Geometry check sheet. Reference: the model listing, model coordinates, mm. Face numbers are marked on the shaded views. A direction names the side the tool comes from. Round coordinates to 2 decimals unless told otherwise and drop trailing zeros. Write each loop counter-clockwise with the first axis right and the second up, starting at its lowest first coordinate (ties: lowest second). Pieces come first, ordered by that corner, then holes. Notation, with made-up numbers: (14, 62) -> (19, 62) arc R25 cw to (19, 88) -> close; hole circle Ø4 at (-11, 49.5). An arc over 180 degrees is marked (long way). Use a Markdown table: item, result.
```python
from build123d import *

# Parameters (mm, degrees)
F0_R          = 14
F1_DEPTH      = 10
F1_DEPTH_BACK = 10
F2_R          = 5
F3_R          = 5
F4_R          = 1
F5_DEPTH      = 25
F6_R          = 5


with BuildPart() as f1:
    # F0 (on Top) → F1 (new body, two sides)
    with BuildSketch(Plane.XY) as f1_sk:
        with BuildLine():
            ThreePointArc((-14.1332940251, -7.5), (3.86440782, -15.5263116097), (16, 0))
            ThreePointArc((16, 0), (3.86440782, 15.5263116097), (-14.1332940251, 7.5))
            ThreePointArc((-14.1332940251, 7.5), (-14.6133919535, 6.5152724896), (-15.0249792013, 5.5))
            ThreePointArc((-15.0249792013, 5.5), (-16, 0), (-15.0249792013, -5.5))
            ThreePointArc((-15.0249792013, -5.5), (-14.6133919535, -6.5152724896), (-14.1332940251, -7.5))
        make_face()
        Circle(F0_R, mode=Mode.SUBTRACT)
        with BuildLine():
            ThreePointArc((-15.0249792013, 5.5), (-14.6133919535, 6.5152724896), (-14.1332940251, 7.5))
            Line((-14.1332940251, 7.5), (-58.6950893998, 7.5))
            Line((-58.6950893998, 7.5), (-58.6950893998, 40))
            Line((-58.6950893998, 40), (-60.6950893998, 40))
            Line((-60.6950893998, 40), (-60.6950893998, -40))
            Line((-60.6950893998, -40), (-58.6950893998, -40))
            Line((-58.6950893998, -40), (-58.6950893998, -7.5))
            Line((-58.6950893998, -7.5), (-14.1332940251, -7.5))
            ThreePointArc((-14.1332940251, -7.5), (-14.6133919535, -6.5152724896), (-15.0249792013, -5.5))
            Line((-15.0249792013, -5.5), (-58.6950893998, -5.5))
            Line((-58.6950893998, -5.5), (-58.6950893998, 5.5))
            Line((-58.6950893998, 5.5), (-15.0249792013, 5.5))
        make_face()
    extrude(amount=F1_DEPTH)
    extrude(f1_sk.sketch, amount=-F1_DEPTH_BACK)

    # F2
    f2_edges = [f1.edges().sort_by_distance(p)[0] for p in [
        (-14.133294, -7.5, 0),
        (-15.024979, -5.5, 0),
        (-15.024979, 5.5, 0),
        (-14.133294, 7.5, 0),
    ]]
    fillet(f2_edges, radius=F2_R)

    # F3
    f3_edges = [f1.edges().sort_by_distance(p)[0] for p in [
        (-58.695089, -5.5, 0),
        (-58.695089, 5.5, 0),
    ]]
    fillet(f3_edges, radius=F3_R)

    # F4 (on face) → F5 (cut)
    with BuildSketch(Plane.XY.offset(10)):
        with Locations((-15.1501176879, -5.7808761485)):
            Circle(F4_R)
        with Locations((-15.2443397102, 5.5276307583)):
            Circle(F4_R)
    extrude(amount=-F5_DEPTH, mode=Mode.SUBTRACT)

    # F6
    f6_edges = [f1.edges().sort_by_distance(p)[0] for p in [
        (-58.695089, 7.5, 0),
    ]]
    fillet(f6_edges, radius=F6_R)


solid = f1.part
```
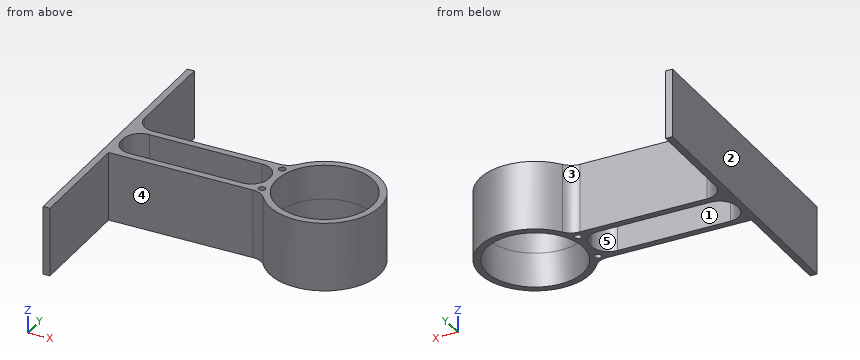
(1) Section check A-A on x = -43. Record the cut outline in (y, z).
A:
| item | result |
|---|---|
| outline | (-7.5, -10) -> (-5.5, -10) -> (-5.5, 10) -> (-7.5, 10) -> close; (5.5, -10) -> (7.5, -10) -> (7.5, 10) -> (5.5, 10) -> close |
(2) Section check C-C on x = -10.5. Record the cut outline in (y, z).
A:
| item | result |
|---|---|
| outline | (-12.07, -10) -> (-9.26, -10) -> (-9.26, 10) -> (-12.07, 10) -> close; (9.26, -10) -> (12.07, -10) -> (12.07, 10) -> (9.26, 10) -> close |
(3) Release check for a two-part mould opening along X. For the marked faces 1 and 2 record: +X half, -X half, draft (parallel to the pull), parting line (faces both ways), or undercut.
A:
| item | result |
|---|---|
| face 1 | undercut |
| face 2 | -X half |
(4) Section check B-B on z = -4. Record the cut outline in (x, y), plus the area to 3 significant figures.
A:
| item | result |
|---|---|
| outline | (-60.7, -40) -> (-58.7, -40) -> (-58.7, -7.5) -> (-16.87, -7.5) arc R5 cw to (-12.86, -9.52) arc R16 ccw (long way) to (-12.86, 9.52) arc R5 cw to (-16.87, 7.5) -> (-53.7, 7.5) arc R5 cw to (-58.7, 12.5) -> (-58.7, 40) -> (-60.7, 40) -> close; hole (-58.7, -0.5) arc R5 ccw to (-53.7, -5.5) -> (-20.99, -5.5) arc R5 ccw to (-16, -0.38) arc R16 cw to (-16, 0.38) arc R5 ccw to (-20.99, 5.5) -> (-53.7, 5.5) arc R5 ccw to (-58.7, 0.5) -> close; hole circle Ø2 at (-15.24, 5.53); hole circle Ø2 at (-15.15, -5.78); hole circle Ø28 at (0, 0) |
| area | 551 mm2 |
(5) Thickness scan on line 1 (Y direction, x = -28, z = 0.5); line 2 (X direction, y = 9.5, z = 7); line 3 (X direction, y = 2, z = 8.5). Record the ranges inside material, lowest first.
A:
| item | result |
|---|---|
| line 1 | y = -7.5 to -5.5, 5.5 to 7.5 |
| line 2 | x = -60.7 to -57.7, -12.87 to -10.28, 10.28 to 12.87 |
| line 3 | x = -60.7 to -58.46, -16.22 to -13.86, 13.86 to 15.87 |
(6) Access from +Z, -Z, +X, -X, +Y, -Y to the whole of each face (thin tool, end or side, straight path). Record for the marked faces 3, 4 and 5.
A:
| item | result |
|---|---|
| face 3 | +Z, -Z, +Y |
| face 4 | +Z, -Z, -Y |
| face 5 | +Z, -Z |
(7) Gauge pin test, flat ends, axial feed: pin 1 Ø12 at (x, z) = (-41, 7.5) entering from +Y; pin 2 Ø2 at (x, z) = (-19, -6.5) entering from -Y; pin 3 Ø1.6 at (x, y) = (-15.15, -5.78) entering from -Z; pin 4 Ø6 at (y, z) = (-28.5, 1.5) entering from +X. Record the tip position at first contact, or that the pin passes through.
A:
| item | result |
|---|---|
| pin 1 | stops at y = 7.5 |
| pin 2 | stops at y = -7.5 |
| pin 3 | passes through |
| pin 4 | stops at x = -58.7 |
